```python
from build123d import *

# Parameters (mm, degrees)
SKETCH1_R            = 3.025
BOSS_EXTRUDE1_DEPTH  = 1.5875
FILLET1_START        = -1
FILLET1_DEPTH        = 4
M4_CLEARANCE_HOLE1_D = 4.5


with BuildPart() as part:
    # Sketch1 → Boss-Extrude1 (new body)
    # profile 1 of 4: a face of its own
    with BuildSketch(Plane(origin=(0, 0, 0), x_dir=(0, 0, -1), z_dir=(1, 0, 0))):
        with BuildLine():
            Line((541.51052412, 64.02688415), (530.217508306, 94.502121028))
            Line((530.217508306, 94.502121028), (516.877503621, 94.502121028))
            Line((516.877503621, 94.502121028), (516.877503621, 59.781603486))
            add(Edge.make_bspline(
                [(516.877503621, 59.781603486), (516.877503621, 66.224434359), (520.85597879, 70.389492112), (525.494944029, 71.935813858)],
                knots=[0.791503971, 0.791503971, 0.791503971, 0.791503971, 1, 1, 1, 1], degree=3, weights=[0.513780637, 0.559932173, 0.722005294, 1]))
            add(Edge.make_bspline(
                [(525.494944029, 71.935813858), (531.367057327, 73.893184958), (538.581630796, 71.930770882), (541.51052412, 64.02688415)],
                knots=[0, 0, 0, 0, 0.245758306, 0.245758306, 0.245758306, 0.245758306], degree=3, weights=[1, 0.672322259, 0.505703571, 0.500143936]))
        make_face()
    # profile 2 of 4: a face of its own
    with BuildSketch(Plane(origin=(0, 0, 0), x_dir=(0, 0, -1), z_dir=(1, 0, 0))):
        with BuildLine():
            Line((516.877503621, 131.502121028), (516.877503621, 94.502121028))
            Line((516.877503621, 94.502121028), (530.217508306, 94.502121028))
            Line((530.217508306, 94.502121028), (530.217508306, 131.502121028))
            ThreePointArc((530.217508306, 131.502121028), (529.222247158, 133.753333946), (526.877503621, 134.502121028))
            Line((526.877503621, 134.502121028), (519.877503621, 134.502121028))
            ThreePointArc((519.877503621, 134.502121028), (517.756183277, 133.623441372), (516.877503621, 131.502121028))
        make_face()
        with Locations((523.717508306, 104.502121028)):
            Circle(SKETCH1_R, mode=Mode.SUBTRACT)
        with Locations((523.717508306, 124.502121028)):
            Circle(SKETCH1_R, mode=Mode.SUBTRACT)
    # profile 3 of 4: a face of its own
    with BuildSketch(Plane(origin=(0, 0, 0), x_dir=(0, 0, -1), z_dir=(1, 0, 0))):
        with Locations((523.717508306, 104.502121028)):
            Circle(SKETCH1_R)
    # profile 4 of 4: a face of its own
    with BuildSketch(Plane(origin=(0, 0, 0), x_dir=(0, 0, -1), z_dir=(1, 0, 0))):
        with Locations((523.717508306, 124.502121028)):
            Circle(SKETCH1_R)
    extrude(amount=BOSS_EXTRUDE1_DEPTH)

    # Fillet1: read off the stored shape, not the designer's step
    # Fillet1 outline → Fillet1 (cut)
    with BuildSketch(Plane.YZ.offset(FILLET1_START)):
        with BuildLine():
            add(Edge.make_bspline(
                [(59.781603486, -516.877503621), (63.745099458, -516.877503621), (67.076255883, -518.543444616), (69.385969927, -521.114832125)],
                knots=[0.791503971, 0.791503971, 0.791503971, 0.791503971, 0.915480845, 0.915480845, 0.915480845, 0.915480845], degree=3, weights=[0.513780637, 0.541223477, 0.609653692, 0.719071281]))
            ThreePointArc((69.385969927, -521.114832125), (68.955807133, -518.383002389), (71.275593157, -516.877503621))
            Line((71.275593157, -516.877503621), (59.781603486, -516.877503621))
        make_face()
        with BuildLine():
            ThreePointArc((74.887594645, -537.485939312), (72.182937452, -536.873853395), (71.650054639, -534.152483223))
            add(Edge.make_bspline(
                [(71.650054639, -534.152483223), (70.307636138, -537.474178056), (67.681794337, -540.156147165), (64.02688415, -541.51052412)],
                knots=[1.132789983, 1.132789983, 1.132789983, 1.132789983, 1.245758306, 1.245758306, 1.245758306, 1.245758306], degree=3, weights=[0.609905504, 0.539286736, 0.502699547, 0.500143936]))
            Line((64.02688415, -541.51052412), (74.887594645, -537.485939312))
        make_face()
    extrude(amount=FILLET1_DEPTH, mode=Mode.SUBTRACT)

    # M4 Clearance Hole1 (through all)
    with Locations(Plane(origin=(1.5875, 0, 0), x_dir=(0, 0, -1), z_dir=(1, 0, 0))):
        with Locations((523.717508306, 124.502121028), (523.717508306, 104.502121028)):
            Hole(M4_CLEARANCE_HOLE1_D / 2)


solid = part.part
```
Geometry check sheet. Reference: the model listing, model coordinates, mm. Coordinates: 2 decimals unless noted, no trailing zeros. Order: outer loops, then holes, each group sorted by start corner. A loop starts at its lowest first (then second) coordinate and runs counter-clockwise, first axis right, second up. Notation, with made-up numbers: M 80.5,-19 L 129.5,-19 A15 ccw 129.5,-5 Z; hole C 80.25,32 d9. An arc over 180 degrees is marked long. Answer as a JSON object with one key per item and string values.
Q1. Scan lines: line 1 (Z direction, x = 0.1, y = 113.5); line 2 (Y direction, x = 1.5, z = -524.75); line 3 (Y direction, x = 1.1, z = -523.75). Record each from-to range of solid material in increasing order.
Results are:
{"line 1": "z = -530.22 to -516.88", "line 2": "y = 71.66 to 102.5, 106.5 to 122.5, 126.5 to 134.5", "line 3": "y = 71.2 to 102.25, 106.75 to 122.25, 126.75 to 134.5"}
Q2. Cross-section at D-D on z = -518. Record the cut outline in (x, y), and give its area (3 significant figures).
Results are:
{"outline": "M 0,69.17 L 1.59,69.17 L 1.59,133.84 L 0,133.84 Z", "area": "103 mm²"}
Q3. Release check for a two-part mould opening along Y. For faces 1 (the cylindrical face through (0.78, 68.94, -518.42)), 2 (the flat face through (1, 134.502, -523)), 3 (the flat face through (1, 113, -530.218)), 4 (the cylindrical face through (0.78, 125.18, -521.57)) record: released by +Y, released by -Y, zero draft, split by the parting line, or undercut.
Results are:
{"face 1": "released by -Y", "face 2": "released by +Y", "face 3": "zero draft", "face 4": "undercut"}
Q4. Depth check by flat-ended pin: pin 1 Ø0.5 at (x, y) = (1, 105.5) entering from -Z. Enter the tip coordinate at first touch or a pass-through.
Results are:
{"pin 1": "stops at z = -530.22"}
Q5. Cross-section at A-A on y = 128.5. Record the cut outline in (x, z), and give its area (3 significant figures).
Results are:
{"outline": "M 0,-530.22 L 1.59,-530.22 L 1.59,-516.88 L 0,-516.88 Z", "area": "21.2 mm²"}
Q6. Cross-section at B-B on z = -522.75. Give the number of separate pieces and of enclosed holes in the cut face, and give its area (3 significant figures).
Results are:
{"separate pieces": "3", "enclosed holes": "0", "area": "88.5 mm²"}
